```python
from build123d import *

# Parameters (mm, degrees)
BASE_EXTRUSION_DEPTH = 19.5
ESQUISSE2_W          = 7
ESQUISSE2_H          = 12
BOSS_EXTRU_1_DEPTH   = 15
CONG_1_R             = 1
ESQUISSE3_W          = 10
ESQUISSE3_H          = 13.5
BOSS_EXTRU_2_DEPTH   = 2
CONG_2_R             = 2


with BuildPart() as part:
    # Esquisse1 → Base-Extrusion (new body)
    with BuildSketch(Plane.XY):
        with BuildLine():
            Line((0, 0), (0, 33))
            ThreePointArc((0, 33), (2, 35), (4, 33))
            Line((4, 33), (4, 0))
            ThreePointArc((4, 0), (2, -2), (0, 0))
        make_face()
    extrude(amount=BASE_EXTRUSION_DEPTH)

    # Esquisse2 → Boss.-Extru.1 (add)
    with BuildSketch(Plane.XY.offset(19.5)):
        with Locations((2, 34)):
            Rectangle(ESQUISSE2_W, ESQUISSE2_H)
    extrude(amount=-BOSS_EXTRU_1_DEPTH)

    # Congé1
    cong_1_edges = [part.edges().sort_by_distance(p)[0] for p in [
        (-1.5, 40, 12),
        (5.5, 40, 12),
    ]]
    fillet(cong_1_edges, radius=CONG_1_R)

    # Esquisse3 → Boss.-Extru.2 (add)
    with BuildSketch(Plane.XY.offset(19.5)):
        with Locations((2, 34.75)):
            Rectangle(ESQUISSE3_W, ESQUISSE3_H)
    extrude(amount=-BOSS_EXTRU_2_DEPTH)

    # Congé2
    cong_2_edges = [part.edges().sort_by_distance(p)[0] for p in [
        (-3, 41.5, 18.5),
        (7, 41.5, 18.5),
    ]]
    fillet(cong_2_edges, radius=CONG_2_R)


solid = part.part
```
Geometry check sheet. Reference: the model listing, model coordinates, mm. A direction names the side the tool comes from. Round coordinates to 2 decimals unless told otherwise and drop trailing zeros. Loops run counter-clockwise (first coordinate to the right, second up) from the corner with the lowest first, then second, coordinate; pieces in that order, holes last. Notation, with made-up numbers: (-27.5, 55.25) -> (15.5, 55.25) arc R24 ccw to (15.5, 79.25) -> close; hole circle Ø4 at (37.25, 8.5). An arc over 180 degrees is marked (long way). Use a Markdown table: item, result.
(1) Sectioned sample at B-B (y = 32). Enter the section's corners in (x, z).
Calculated:
| item | result |
|---|---|
| outline | (-3, 17.5) -> (-1.5, 17.5) -> (-1.5, 4.5) -> (0, 4.5) -> (0, 0) -> (4, 0) -> (4, 4.5) -> (5.5, 4.5) -> (5.5, 17.5) -> (7, 17.5) -> (7, 19.5) -> (-3, 19.5) -> close |
(2) Sectioned sample at C-C (z = 6.25). Enter the section's corners in (x, y), then the cut area to 3 significant figures.
Calculated:
| item | result |
|---|---|
| outline | (-1.5, 28) -> (0, 28) -> (0, 0) arc R2 ccw to (4, 0) -> (4, 28) -> (5.5, 28) -> (5.5, 39) arc R1 ccw to (4.5, 40) -> (-0.5, 40) arc R1 ccw to (-1.5, 39) -> close |
| area | 202 mm² |
(3) Set-up check for faces 1 (the flat face through (5.5, 33, 11)), 2 (the cylindrical face through (2, 35, 2)), 3 (the cylindrical face through (5.199, 39.715, 10.909)), 4 (the flat face through (5, 28, 12)): record each of +Z, -Z, +X, -X, +Y, -Y from which the full face is reachable in a straight line by a thin tool's end or side.
Calculated:
| item | result |
|---|---|
| face 1 | -Z, +X, +Y, -Y |
| face 2 | -Z, +Y |
| face 3 | -Z, +X, +Y |
| face 4 | +Z, -Z, +X, -Y |
(4) Sectioned sample at A-A (x = 2). Enter the section's corners in (y, z).
Calculated:
| item | result |
|---|---|
| outline | (-2, 0) -> (35, 0) -> (35, 4.5) -> (40, 4.5) -> (40, 17.5) -> (41.5, 17.5) -> (41.5, 19.5) -> (-2, 19.5) -> close |
(5) Sectioned sample at D-D (y = 19.5). Enter the section's corners in (x, z), then the cut area to 3 significant figures.
Calculated:
| item | result |
|---|---|
| outline | (0, 0) -> (4, 0) -> (4, 19.5) -> (0, 19.5) -> close |
| area | 78.0 mm² |
(6) Scan lines: probe 1 along Y at (x, z) = (-0.25, 10.75); probe 2 along X at (y, z) = (6.5, 18); probe 3 along X at (y, z) = (33, 7.5). Record each from-to range of solid material in increasing order.
Calculated:
| item | result |
|---|---|
| probe 1 | 28 to 40 |
| probe 2 | 0 to 4 |
| probe 3 | -1.5 to 5.5 |
(7) Go/stop test with flat-tipped pins: P1, Ø6, axis at y = 27, z = 13, coming from the +X side; P2, Ø10, axis at y = 21, z = 10.5, coming from the -X side; P3, Ø6, axis at x = 4, z = 4, coming from the +Y side; P4, Ø2, axis at x = 3.5, y = 35, coming from the -Z side. Record where each tip stops, or that it passes through.
Calculated:
| item | result |
|---|---|
| P1 | x = 5.5 |
| P2 | x = 0 |
| P3 | y = 40 |
| P4 | z = 0 |
